Autodesk Inventor part; units mm, degrees
ref_plane "YZ Plane" through (0, 0, 0) normal (1, 0, 0) x (0, 1, 0)
ref_plane "XZ Plane" through (0, 0, 0) normal (0, 1, 0) x (-1, 0, 0)
ref_plane "XY Plane" through (0, 0, 0) normal (0, 0, 1) x (1, 0, 0)
ref_plane "Work Plane3" through (42.3, -5.3, -4.5) normal (1, 0, 0) x (0, 1, 0)
sketch "Sketch3" plane through (42.3, -5.3, -4.5) normal (1, 0, 0) x (0, 1, 0)
  line L0 (3.5, 2.5) -> (6, 0)
  line L1 (6, -5) -> (6, 0)
  line L2 (3.5, 2.5) -> (21.8, 2.5)
  line L3 (6, -5) -> (21.8, -5)
  line L4 (21.8, -5) -> (21.8, 2.5)
  line L5 (21.7, 2.4) -> (21.7, -4.9)
  line L6 (21.7, -4.9) -> (6.1, -4.9)
  line L7 (6.1, -4.9) -> (6.1, 0.0414)
  line L8 (6.1, 0.0414) -> (3.7414, 2.4)
  line L9 (3.7414, 2.4) -> (21.7, 2.4)
  point P0 (21.7, 2.4)
  dimension "d0" = 0.1
  dimension "d36" = 15.8
  dimension "d37" = 7.3
  dimension "d38" = 15.7
  dimension "d39" = 15.7
  dimension "d40" = 12.7986
extrude "Extrusion1" add sketch "Sketch3" against normal blind 75 contours L5 L6 L7 L8 L9
sketch "Sketch4" plane through (42.3, 16.4, -2.1) normal (0, 1, 0) x (1, 0, 0)
  line L0 (-60, -0.1) -> (-75, -0.1)
  line L1 (-75, -0.1) -> (-75, -7.1)
  line L2 (-60, 0) -> (-75, 0)
  line L3 (-75, 7.3) -> (-60, 7.3)
  arc A0 (-75, -7.1) -> (-70, -12.1) centre (-70, -7.1) ccw
  line L4 (-60, -12.1) -> (-70, -12.1)
  line L5 (-60, -0.1) -> (-60, -8.7171)
  line L6 (-60, -10.4829) -> (-60, -12.1)
  line L7 (-60, -10.4829) -> (-63.5, -11.1)
  line L8 (-63.5, -11.1) -> (-63.5, -8.1)
  line L9 (-63.5, -8.1) -> (-60, -8.7171)
  line L10 (-60, 0) -> (-60, 7.3)
  line L11 (-75, 0) -> (-75, 7.3)
  dimension "d41" = 15
extrude "Extrusion2" add sketch "Sketch4" along normal blind 50 contours L2 L11 L3 L10
sketch "Sketch5" plane through (-32.7, -5.3, -4.5) normal (-1, 0, 0) x (0, 0, 1)
  line L0 (2.4, 3.7414) -> (2.4, 71.7)
  line L1 (2.4, 71.7) -> (2.4, 3.7414)
  line L2 (-4.9, 6.1) -> (0.0414, 6.1)
  line L3 (2.4, 3.7414) -> (0.0414, 6.1)
  line L4 (0.0414, 6.1) -> (-4.9, 6.1)
  line L5 (2.4, 71.7) -> (-4.9, 6.1)
  line L6 (2.4, 71.7) -> (-4.9, 71.7)
  line L7 (-4.9, 71.7) -> (-4.9, 6.1)
extrude "Extrusion3" cut sketch "Sketch5" against normal through all contours L5 L7 L6
sketch "Sketch6" plane through (42.3, -5.3, -4.5) normal (1, 0, 0) x (0, 0, -1)
  line L0 (3.164, 21.7) -> (-2.4, 71.7)
  line L1 (4.9, 6.1) -> (3.164, 21.7)
  line L2 (3.164, 21.7) -> (-2.4, 21.7)
  line L3 (-2.4, 3.7414) -> (-2.4, 71.7)
  line L4 (4.9, 6.1) -> (-2.4, 21.7)
extrude "Extrusion4" cut sketch "Sketch6" against normal blind 60 contours L1 L4 L2
sketch "Sketch7" plane through (-32.7, -1.5586, -2.1) normal (0, 0, 1) x (1, 0, 0)
  line L0 (75, 0) -> (0, 0)
  line L1 (0, 0) -> (0, 67.9586)
  line L2 (0, 67.9586) -> (15, 67.9586)
  line L3 (15, 17.9586) -> (15, 67.9586)
  point P0 (32.7, 1.5586)
  point P1 (37.5, 8.5)
  point P2 (7.5, 33.9793)
  point P3 (15, 22.6774)
  dimension "d10" = 37.5
  dimension "d11" = 8.5
  dimension "d12" = 7.5
  dimension "d13" = 33.9793
hole "Hole1" at (4.8, 6.9414, -2.1) at (-25.2, 32.4207, -2.1) direction (0, 0, -1) diameter 3.4 end through all
ref_plane "Work Plane4" through (-32.7, -1.5586, -5.35) normal (0, 0, 1) x (1, 0, 0)
sketch "Sketch10" plane through (-32.7, -1.5586, -5.35) normal (0, 0, 1) x (1, 0, 0)
  point P0 (32.7, 1.5586)
  point P1 (37.5, 8.5)
  point P2 (7.5, 33.9793)
hole "Hole2" at (4.8, 6.9414, -5.35) at (-25.2, 32.4207, -5.35) direction (0, 0, -1) diameter 6 end through all
fillet "Fillet2" radius 2 1 edges at (-17.7, 8.6, -5.75)
properties part number "Base Gripper Support"
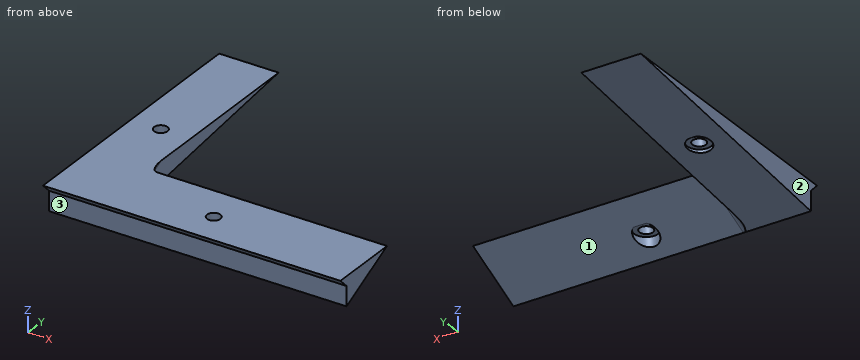
Read the model definition and answer for the solid it produces. Units are mm, in the model's axes. Face numbers are marked on the shaded views. A direction names the side the tool comes from. Round coordinates to 2 decimals unless told otherwise and drop trailing zeros. Write each loop counter-clockwise with the first axis right and the second up, starting at its lowest first coordinate (ties: lowest second). Pieces come first, ordered by that corner, then holes. Notation, with made-up numbers: M 31,-1 L 56,-1 A18 cw 56,34 Z; hole C 57,23.25 d5. An arc over 180 degrees is marked long. Use a Markdown table: item, result.
1) Straight lines are drawn through the part: line 1 along X through (y, z) = (35, -4.25); line 2 along Y through (x, z) = (4.8, -6.25); line 3 along Z through (x, y) = (-1, 12.5) (3 decimals). For each, find the intervals that lie inside material, in ascending order. Write a range as [from, to].
Answers follow:
| item | result |
|---|---|
| line 1 | x = [-32.7, -17.7] |
| line 2 | y = [0.8, 3.94] |
| line 3 | z = [-3.925, -2.1] |
2) The part is cut by section A-A (x = 4.8). Write down the section's boundary in (y, z).
Answers follow:
| item | result |
|---|---|
| outline | M -1.56,-2.1 L 0.8,-4.46 L 0.8,-9.4 L 3.94,-7.93 L 3.94,-5.35 L 5.24,-5.35 L 5.24,-2.1 Z; M 8.64,-5.35 L 9.45,-5.35 L 16.4,-2.1 L 8.64,-2.1 Z |
3) The part is cut by section D-D (x = -3). Write down the section's boundary in (y, z).
Answers follow:
| item | result |
|---|---|
| outline | M -1.56,-2.1 L 0.8,-4.46 L 0.8,-9.4 L 16.4,-2.1 Z |
4) A tool of negligible diameter and unlimited length cuts with its end or side. For the marked faces 1, 2 and 3, from which of +Z, -Z, +X, -X, +Y, -Y can it reach the whole face along a straight path? Write none if from no direction.
Answers follow:
| item | result |
|---|---|
| face 1 | -Z, +X, +Y |
| face 2 | +Z, -Z, -X, +Y, -Y |
| face 3 | -Z, +X, -X, -Y |
5) Flat-ended cylindrical pins translate along their axes: pin 1 (4 mm diameter, centred on x = 1.5, z = -7.5, fed in from -Y); pin 2 (8 mm diameter, centred on x = 4.8, y = 6.94, fed in from +Z); pin 3 (4.5 mm diameter, centred on x = 5, y = 5.5, fed in from -Z); pin 4 (2 mm diameter, centred on x = -9.5, z = -6, fed in from +Y). Find the tip coordinate at first contact, or state that the pin passes through.
Answers follow:
| item | result |
|---|---|
| pin 1 | stops at y = 0.8 |
| pin 2 | stops at z = -2.1 |
| pin 3 | stops at z = -8.25 |
| pin 4 | stops at y = 10.2 |
6) The part is cut by section B-B (x = -25.2). Write down the section's boundary in (y, z).
Answers follow:
| item | result |
|---|---|
| outline | M -1.56,-2.1 L 0.8,-4.46 L 0.8,-9.4 L 29.42,-6.22 L 29.42,-5.35 L 30.72,-5.35 L 30.72,-2.1 Z; M 34.12,-5.35 L 35.42,-5.35 L 35.42,-5.55 L 66.4,-2.1 L 34.12,-2.1 Z |
7) The part is cut by section C-C (y = 45.5). Write down the section's boundary in (x, z).
Answers follow:
| item | result |
|---|---|
| outline | M -32.7,-4.43 L -17.7,-4.43 L -17.7,-2.1 L -32.7,-2.1 Z |
